from build123d import *

# Parameters (mm, degrees)
SKETCH10_R         = 2.291358881
CUT_EXTRUDE2_DEPTH = 2.0447
CUT_EXTRUDE2_TAPER = 45
CUT_EXTRUDE1_DEPTH = 2.0447


with BuildPart() as part:
    # Sketch11 → Revolve1 (revolve)
    with BuildSketch(Plane(origin=(0, 0, 0), x_dir=(0, 0, -1), z_dir=(1, 0, 0))):
        with BuildLine():
            Line((-7.855712, 6.7437), (-3.8481, 3.259936038))
            ThreePointArc((-3.8481, 3.259936038), (-3.742193592, 3.196928347), (-3.620928247, 3.175))
            Line((-3.620928247, 3.175), (6.985, 3.175))
            Line((6.985, 3.175), (7.9375, 2.2225))
            Line((7.9375, 2.2225), (7.9375, 0))
            Line((7.9375, 0), (-7.9375, 0))
            Line((-7.9375, 0), (-7.9375, 6.7437))
            Line((-7.9375, 6.7437), (-7.855712, 6.7437))
        make_face()
    revolve(axis=Axis((0, 0, -7.9375), (0, 0, 1)))

    # Sketch10 → Cut-Extrude2 (cut)
    with BuildSketch(Plane.XY.offset(7.9375)):
        Circle(SKETCH10_R)
    extrude(amount=-CUT_EXTRUDE2_DEPTH, taper=CUT_EXTRUDE2_TAPER, mode=Mode.SUBTRACT)

    # Sketch9 → Cut-Extrude1 (cut)
    with BuildSketch(Plane.XY.offset(7.9375)):
        Polygon((1.984375, -1.14567944), (1.984375, 1.14567944), (0, 2.291358881), (-1.984375, 1.14567944), (-1.984375, -1.14567944), (0, -2.291358881), align=None)
    extrude(amount=-CUT_EXTRUDE1_DEPTH, mode=Mode.SUBTRACT)


solid = part.part
Source: CAD feature listing. Evaluate the final solid. Frame: model axes, mm. A direction names the side the tool comes from. Give positions to 0.01 mm unless a question says otherwise; leave off trailing zeros. Write each loop counter-clockwise with the first axis right and the second up, starting at its lowest first coordinate (ties: lowest second). Pieces come first, ordered by that corner, then holes. Notation, with made-up numbers: M 31.25,66 L 89.25,66 A7 ccw 89.25,72 Z; hole C 70.5,-11.5 d8. An arc over 180 degrees is marked long. Answer as a JSON object with one key per item and string values.
Q1. Cut plane B-B, the plane z = 2. Return the cut outline in (x, y) (3 decimals).
Geometry check:
{"outline": "C 0,0 d6.35"}
Q2. Access query for faces 4 (the face through (1.08, 1.84, 7.78)), 5 (the face through (3.348, -0.743, 4.043)). Directions: +Z, -Z, +X, -X, +Y, -Y. A direction counts if a zero-diameter tool reaches every point of the face in a straight line with its end or side. Return the directions, or none.
Geometry check:
{"face 4": "+Z", "face 5": "-Z"}
Q3. Mould query, pull axis Y, two halves, no side actions, for faces 1 (the face through (3.1, -0.69, -1.76)), 2 (the face through (1.984, 0, 7)), 3 (the face through (0, -3, 7.938)). Classes: +Y half, -Y half, draft (parallel to the pull), parting line (faces both ways), or undercut.
Geometry check:
{"face 1": "parting line", "face 2": "undercut", "face 3": "draft"}
Q4. Contact query for flat-ended pins moving along their axis: P1, Ø8, axis at x = 3, z = 0.5, coming from the +Y side; P2, Ø1, axis at y = 0.5, z = 7, coming from the -X side; P3, Ø2, axis at y = 0, z = 7, coming from the +X side; P4, Ø1, axis at x = -4, y = 3, coming from the -Z side. Output: stop coordinate, or through.
Geometry check:
{"P1": "stops at y = 3.25", "P2": "stops at x = -6.42", "P3": "stops at x = 6.74", "P4": "stops at z = 5.27"}
Q5. Ray query, line 1 along Z through (x, y) = (0.75, 0.5); line 2 along X through (y, z) = (0, 0) (3 decimals); line 3 along Y through (x, z) = (-2, 0.75). Return the intervals inside material, ascending.
Geometry check:
{"line 1": "z = -7.94 to 5.89", "line 2": "x = -3.175 to 3.175", "line 3": "y = -2.47 to 2.47"}
